from build123d import *

# Parameters (mm, degrees)
F0_W     = 482.6
F0_H     = 812.8
F1_DEPTH = 482.6
F2_W     = 355.6
F2_H     = 355.6
F3_DEPTH = 50.8
F2_W_2   = 431.8
F2_H_2   = 431.8
F4_DEPTH = 25.4


with BuildPart() as f1:
    # F0 (on Top) → F1 (new body)
    with BuildSketch(Plane.XY):
        with Locations((-446.823381, -61.770858)):
            Rectangle(F0_W, F0_H)
    extrude(amount=F1_DEPTH)

    # F2 (on face) → F3 (join)
    with BuildSketch(Plane(origin=(0, 344.629142, 0), x_dir=(-1, 0, 0), z_dir=(0, 1, 0))):
        with Locations((446.823381, 241.3)):
            Rectangle(F2_W, F2_H)
    extrude(amount=F3_DEPTH)

    # F2 (on face) → F4 (join)
    with BuildSketch(Plane(origin=(0, 344.629142, 0), x_dir=(-1, 0, 0), z_dir=(0, 1, 0))):
        with Locations((446.823381, 241.3)):
            Rectangle(F2_W_2, F2_H_2)
        with Locations((446.823381, 241.3)):
            Rectangle(F2_W, F2_H, mode=Mode.SUBTRACT)
    extrude(amount=F4_DEPTH)


solid = f1.part
Verification items for the finished model (mm, model axes). A direction names the side the tool comes from. Give positions to 0.01 mm unless a question says otherwise; leave off trailing zeros. Use CSV: the item, a comma, the result in double quotes.
(1) Set-up check for faces 1 (the flat face through (-205.523, -67, 238)), 2 (the flat face through (-444, 357, 457.2)), 3 (the flat face through (-444, 383, 63.5)), 4 (the flat face through (-662.723, 357, 238)), 5 (the flat face through (-269.023, 383, 239)): record each of +Z, -Z, +X, -X, +Y, -Y from which the full face is reachable in a straight line by a thin tool's end or side.
Derived:
face 1,"+Z, -Z, +X, +Y, -Y"
face 2,"+Z, +X, -X, +Y"
face 3,"-Z, +X, -X, +Y"
face 4,"+Z, -Z, -X, +Y"
face 5,"+Z, -Z, +X, +Y"
(2) Go/stop test with flat-tipped pins: pin 1 (20.5 mm diameter, centred on y = 383.5, z = 271.5, fed in from +X); pin 2 (12.5 mm diameter, centred on y = 357, z = 235.5, fed in from -X); pin 3 (12.5 mm diameter, centred on x = -474.5, y = 378, fed in from -Z). Record where each tip stops, or that it passes through.
Derived:
pin 1,"stops at x = -269.02"
pin 2,"stops at x = -662.72"
pin 3,"stops at z = 63.5"
(3) Material ranges on L1, parallel to Y at x = -657, z = 306, recorded low to high.
Derived:
L1,"y = -468.17 to 370.03"
